```python
from build123d import *

# Parameters (mm, degrees)
SKETCH_W     = 40.3
SKETCH_H     = 19.5
PAD_DEPTH    = 35
SKETCH001_R  = 2.9
PAD001_DEPTH = 43


with BuildPart() as part:
    # Sketch → Pad (new body)
    with BuildSketch(Plane.XY):
        Rectangle(SKETCH_W, SKETCH_H)
    extrude(amount=PAD_DEPTH)

    # Sketch001 → Pad001 (join)
    with BuildSketch(Plane.XY):
        with Locations((6.425, 0)):
            Circle(SKETCH001_R)
    extrude(amount=PAD001_DEPTH)


solid = part.part
```
The listing builds one solid part. Answer for the finished solid, in the listing's coordinates (mm). Round coordinates to 2 decimals unless told otherwise and drop trailing zeros. Loops run counter-clockwise (first coordinate to the right, second up) from the corner with the lowest first, then second, coordinate; pieces in that order, holes last. Notation, with made-up numbers: (5, -20) - (19, -20) arc R19 cw to (19, 13) - close; hole circle Ø9 at (-7.75, 65.5). An arc over 180 degrees is marked (long way). Use one line per item in the form item = value. Start each with the question number.
1. For a pull along Z with two mould halves and no side action, classify faces 1 (the face through (0, 0, 35)), 2 (the face through (0, 0, 0)), 3 (the face through (9.104, -1.111, 38.944)) as pulls with the +Z half, pulls with the -Z half, needs draft (parallel to the pull), parting line crosses it, or undercut.
2. The part is cut by section A-A on y = 0. Determine the outline of the cut face in (x, z) (3 decimals), then the cut area to 3 significant figures.
3. Consider line 1 (Z direction, x = 0, y = 2.75); line 2 (X direction, y = -1.75, z = 36). Determine where each line is inside the solid, lowest interval first. Write a range as [from, to].
4. The part is cut by section B-B on x = -13.5. Determine the outline of the cut face in (y, z).
5. The part is cut by section C-C on y = 2.25. Determine the outline of the cut face in (x, z), then the cut area to 3 significant figures.
Geometry check:
q1.face_1 = pulls with the +Z half
q1.face_2 = pulls with the -Z half
q1.face_3 = needs draft
q2.outline = (-20.15, 0) - (20.15, 0) - (20.15, 35) - (9.325, 35) - (9.325, 43) - (3.525, 43) - (3.525, 35) - (-20.15, 35) - close
q2.area = 1,460 mm^2
q3.line_1 = [0, 35]
q3.line_2 = [4.11, 8.74]
q4.outline = (-9.75, 0) - (9.75, 0) - (9.75, 35) - (-9.75, 35) - close
q5.outline = (-20.15, 0) - (20.15, 0) - (20.15, 35) - (8.25, 35) - (8.25, 43) - (4.6, 43) - (4.6, 35) - (-20.15, 35) - close
q5.area = 1,440 mm^2
